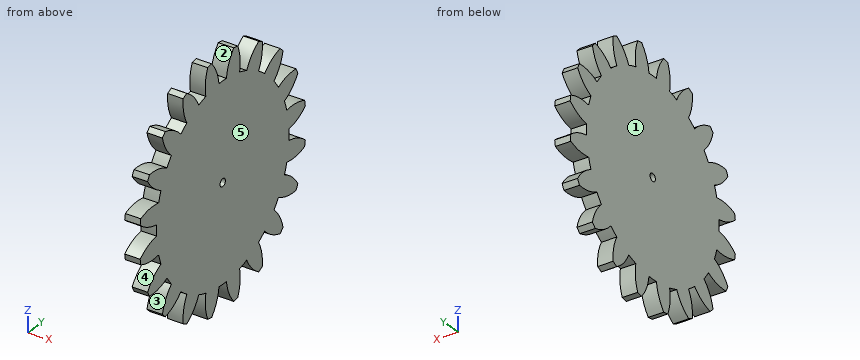
from build123d import *

# Parameters (mm, degrees)
BASPROSKE_W         = 30
BASPROSKE_H         = 55
TOOTHCUT_DEPTH      = 84.366660003
TEETHCUTS_COUNT     = 20
TEETHCUTS_ANGLE     = 342
HUBNEABOTSKE_R      = 12.5
HUBNEARBOTH_DEPTH   = 5.0000254
HUBFAR_START        = 5.0000254
HUBFARSKE_R         = 12.5
HUBFAR_DEPTH        = 5.0000254
BORSKE_R            = 5
BORE_DEPTH          = 40.0000508
SKETCH1_R           = 7
SKETCH1_R_2         = 1.75
BOSS_EXTRUDE1_DEPTH = 40.0000508
SKETCH2_R           = 61.585306659
CUT_EXTRUDE1_DEPTH  = 28
SKETCH3_R           = 13.575984162
CUT_EXTRUDE4_DEPTH  = 5.0000254


with BuildPart() as part:
    # BasProSke → Base-Revolve (revolve)
    with BuildSketch(Plane(origin=(0, 0, 0), x_dir=(1, 0, 0), z_dir=(0, 1, 0)), mode=Mode.PRIVATE) as base_revolve_sk:
        with Locations((15, 27.5)):
            Rectangle(BASPROSKE_W, BASPROSKE_H)
    revolve(base_revolve_sk.sketch.rotate(Axis((-10, 0, 0), (1, 0, 0)), 180), axis=Axis((-10, 0, 0), (1, 0, 0)))

    # TooCutSke → ToothCut (cut, through all)
    with BuildSketch(Plane(origin=(0, 0, 0), x_dir=(0, 0, -1), z_dir=(1, 0, 0))):
        with BuildLine():
            ThreePointArc((2.464838288, 43.679509764), (0, 43.749), (-2.464838288, 43.679509764))
            ThreePointArc((-2.464838288, 43.679509764), (-4.057398861, 49.476814676), (-7.300899231, 54.538899105))
            ThreePointArc((-7.300899231, 54.538899105), (0, 55.0254), (7.300899231, 54.538899105))
            ThreePointArc((7.300899231, 54.538899105), (4.057398861, 49.476814676), (2.464838288, 43.679509764))
        make_face()
    toothcut = extrude(amount=TOOTHCUT_DEPTH, mode=Mode.SUBTRACT)

    # TeethCuts: ToothCut ×20 about axis
    teethcuts_axis = Axis((-10, 0, 0), (1, 0, 0))
    for i in range(1, TEETHCUTS_COUNT):
        add(toothcut.rotate(teethcuts_axis, i * TEETHCUTS_ANGLE / (TEETHCUTS_COUNT - 1)), mode=Mode.SUBTRACT)

    # HubNeaBotSke → HubNearBoth (add)
    with BuildSketch(Plane.ZY):
        with Locations(Location((0, 0, 0), (0, 0, 180))):
            Circle(HUBNEABOTSKE_R)
    extrude(amount=HUBNEARBOTH_DEPTH)

    # HubFarSke → HubFar (add)
    with BuildSketch(Plane(origin=(30, 0, 0), x_dir=(0, 0, -1), z_dir=(1, 0, 0)).offset(HUBFAR_START)):
        Circle(HUBFARSKE_R)
    extrude(amount=-HUBFAR_DEPTH)

    # BorSke → Bore (cut, symmetric)
    with BuildSketch(Plane(origin=(0, 0, 0), x_dir=(0, 0, -1), z_dir=(1, 0, 0))):
        with Locations(Location((0, 0, 0), (0, 0, 180))):
            Circle(BORSKE_R)
    extrude(amount=BORE_DEPTH, both=True, mode=Mode.SUBTRACT)

    # Sketch1 → Boss-Extrude1 (add)
    with BuildSketch(Plane.ZY.offset(5.0000254)):
        Circle(SKETCH1_R)
        Circle(SKETCH1_R_2, mode=Mode.SUBTRACT)
    extrude(amount=-BOSS_EXTRUDE1_DEPTH)

    # Sketch2 → Cut-Extrude1 (cut)
    with BuildSketch(Plane(origin=(35.0000254, 0, 0), x_dir=(0, 0, -1), z_dir=(1, 0, 0))):
        Circle(SKETCH2_R)
    extrude(amount=-CUT_EXTRUDE1_DEPTH, mode=Mode.SUBTRACT)

    # Sketch3 → Cut-Extrude4 (cut)
    with BuildSketch(Plane.ZY.offset(5.0000254)):
        Circle(SKETCH3_R)
    extrude(amount=-CUT_EXTRUDE4_DEPTH, mode=Mode.SUBTRACT)


solid = part.part
Design review of the part built by this model. Coordinates are the model's own, in mm. Face numbers are marked on the shaded views. A direction names the side the tool comes from. Coordinates: 2 decimals unless noted, no trailing zeros. Write each loop counter-clockwise with the first axis right and the second up, starting at its lowest first coordinate (ties: lowest second). Pieces come first, ordered by that corner, then holes. Notation, with made-up numbers: (59.25, 4.25) - (115.25, 4.25) arc R37 ccw to (115.25, 41.25) - close; hole circle Ø6 at (-30, 77.5). An arc over 180 degrees is marked (long way). One line per item, written item: value.
1) For the marked faces 4 and 5, list the 3-axis set-ups (+Z, -Z, +X, -X, +Y, -Y) from which the entire face can be reached by the end or side of a thin tool; tool diameter is ignored.
Answer sheet:
face 4: +X, -X, -Y
face 5: +Z, -Z, +X, +Y, -Y
2) Mouldability with a two-part tool opening along Z and no side actions: class the marked faces 1, 2 and 3 as +Z half, -Z half, draft (parallel to the pull), parting line (faces both ways), or undercut.
Answer sheet:
face 1: draft
face 2: +Z half
face 3: undercut
3) Add section C-C (y = 46.5). State the section outline as (x, z) points.
Answer sheet:
outline: (0, -26.24) - (7, -26.24) - (7, -19.81) - (0, -19.81) - close; (0, -11.54) - (7, -11.54) - (7, -3) - (0, -3) - close; (0, 3) - (7, 3) - (7, 11.54) - (0, 11.54) - close; (0, 19.81) - (7, 19.81) - (7, 26.24) - (0, 26.24) - close
4) Add section D-D (y = 14). State the section outline as (x, z) points, plus the area to 3 significant figures.
Answer sheet:
outline: (0, -41.45) - (7, -41.45) - (7, 41.45) - (0, 41.45) - close
area: 580 mm2
5) To check wall thickness, follow probe 1 along Z at (x, y) = (1.75, -38); probe 2 along Z at (x, y) = (5.5, -22); probe 3 along Z at (x, y) = (1, 1.5). State the ranges of each line that lie inside material, in increasing order.
Answer sheet:
probe 1: z = -39.76 to -33.01, -24.31 to 24.31, 33.01 to 39.76
probe 2: z = -48.41 to 48.41
probe 3: z = -43.72 to -0.9, 0.9 to 43.72
6) Add section A-A (z = 0). State the section outline as (x, y) points.
Answer sheet:
outline: (0, -43.75) - (7, -43.75) - (7, -1.75) - (0, -1.75) - close; (0, 1.75) - (7, 1.75) - (7, 43.75) - (0, 43.75) - close
7) Insertion check: pin 1 (1.5 mm diameter, centred on x = 2, y = 22.5, fed in from -Z); pin 2 (2 mm diameter, centred on x = 5, z = -42.5, fed in from -Y); pin 3 (4 mm diameter, centred on x = 2.5, z = -17, fed in from -Y). Each pin has a flat end and moves straight along its axis. Give the tip position at first contact, or say it passes through.
Answer sheet:
pin 1: stops at z = -49.28
pin 2: stops at y = -26
pin 3: stops at y = -45.64
